Drawing for the job (mm, zero at the part's lowest x, y, z). Round coordinates to 2 decimals unless told otherwise and drop trailing zeros. Loops run counter-clockwise (first coordinate to the right, second up) from the corner with the lowest first, then second, coordinate; pieces in that order, holes last. Notation, with made-up numbers: (-8.75, 3) - (44.25, 3) arc R21 ccw to (44.25, 29) - close; hole circle Ø5 at (-30.5, -12.5). An arc over 180 degrees is marked (long way). Put each result on its own line as item: value.
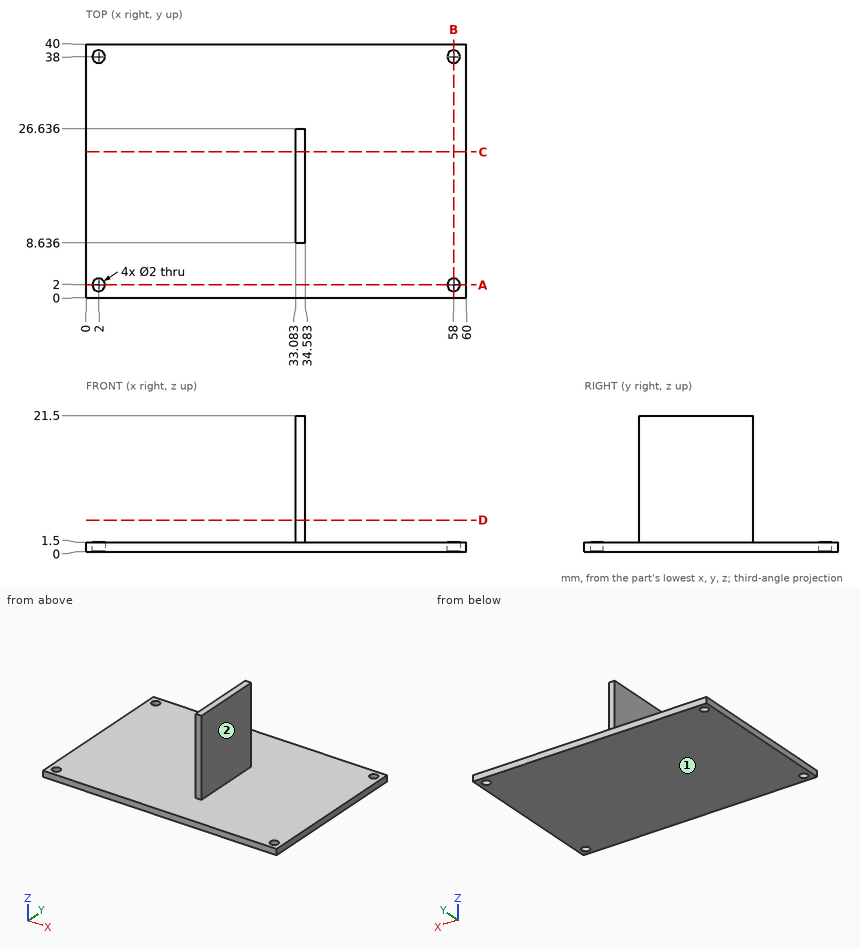
1. Band-saw the part on B-B (x = 58). List the corners of the cut face in (y, z).
A:
outline: (0, 0) - (1, 0) - (1, 1.5) - (0, 1.5) - close; (3, 0) - (37, 0) - (37, 1.5) - (3, 1.5) - close; (39, 0) - (40, 0) - (40, 1.5) - (39, 1.5) - close
2. Band-saw the part on D-D (z = 5). List the corners of the cut face in (x, y) (1 decimal).
A:
outline: (33.1, 8.6) - (34.6, 8.6) - (34.6, 26.6) - (33.1, 26.6) - close
3. Pin check, flat tips, straight feed: P1, Ø4, axis at x = 31, z = 8, coming from the -Y side; P2, Ø5, axis at x = 45.5, y = 17.5, coming from the -Z side; P3, Ø1.6, axis at x = 34, z = 16, coming from the +Y side; P4, Ø12, axis at y = 14.5, z = 8, coming from the +X side. Stop position of each tip, or through.
A:
P1: passes through
P2: stops at z = 0
P3: stops at y = 26.64
P4: stops at x = 34.58
4. Two-plate mould, pull along Z, no slides. Class the marked faces 1 and 2: pulls with the +Z half, pulls with the -Z half, needs draft (parallel to the pull), parting line crosses it, or undercut.
A:
face 1: pulls with the -Z half
face 2: needs draft
5. Probe line 1 along Y through (x, z) = (2, 1); line 2 along X through (y, z) = (38, 1.2); line 3 along Z through (x, y) = (46, 21.5). List the from-to ranges inside material, lowest first. Write a range as [from, to].
A:
line 1: y = [0, 1], [3, 37], [39, 40]
line 2: x = [0, 1], [3, 57], [59, 60]
line 3: z = [0, 1.5]
6. Band-saw the part on C-C (y = 23). List the corners of the cut face in (x, z), plus the area to 3 significant figures.
A:
outline: (0, 0) - (60, 0) - (60, 1.5) - (34.58, 1.5) - (34.58, 21.5) - (33.08, 21.5) - (33.08, 1.5) - (0, 1.5) - close
area: 120 mm²
7. Band-saw the part on A-A (y = 2). List the corners of the cut face in (x, z).
A:
outline: (0, 0) - (1, 0) - (1, 1.5) - (0, 1.5) - close; (3, 0) - (57, 0) - (57, 1.5) - (3, 1.5) - close; (59, 0) - (60, 0) - (60, 1.5) - (59, 1.5) - close
